Source: three-view drawing plus pictorial views. Frame: mm from the lowest corner of the part. Round coordinates to 2 decimals unless told otherwise and drop trailing zeros. Write each loop counter-clockwise with the first axis right and the second up, starting at its lowest first coordinate (ties: lowest second). Pieces come first, ordered by that corner, then holes. Notation, with made-up numbers: M 31.5,42 L 61.5,42 A21 ccw 61.5,54 Z; hole C 4,7.5 d4. An arc over 180 degrees is marked long. Put each result on its own line as item: value. Start each with the question number.
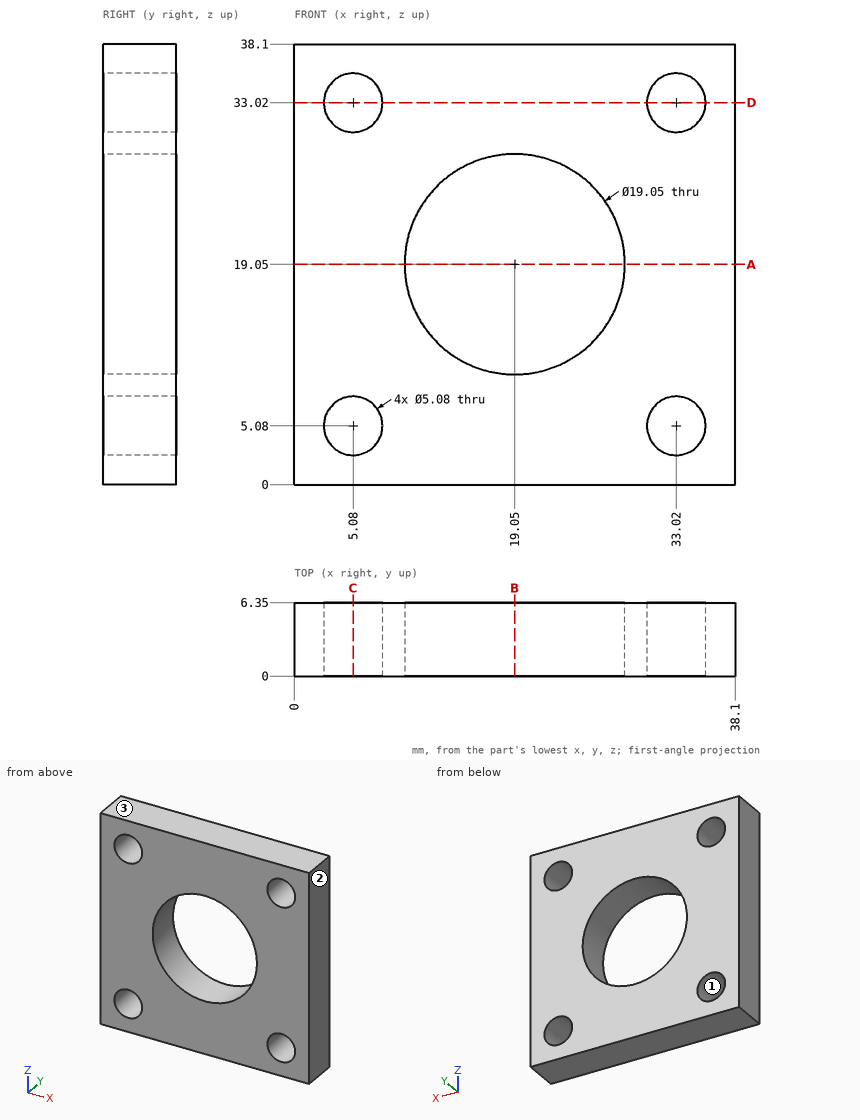
(1) Section query B-B (x = 19.05). Return loops of the section in (y, z) (3 decimals).
(2) Pull-direction query (X, two-part tool) for the marked faces 1, 2 and 3; classes: +X half, -X half, draft (parallel to the pull), parting line (faces both ways), or undercut.
(3) Section query C-C (x = 5.08). Return loops of the section in (y, z), and give its area (3 significant figures).
(4) Contact query for a flat-ended pin moving along its axis: P1, Ø8, axis at x = 16, z = 18, coming from the +Y side. Output: stop coordinate, or through.
(5) Ray query, line 1 along Z through (x, y) = (5.08, 3.75); line 2 along X through (y, z) = (1, 19.5). Return the intervals inside material, ascending.
(6) Section query A-A (z = 19.05). Return loops of the section in (x, y) (3 decimals), and give its area (3 significant figures).
(7) Section query D-D (z = 33.02). Return loops of the section in (x, y), and give its area (3 significant figures).
Entries:
1. outline: M 0,0 L 6.35,0 L 6.35,9.525 L 0,9.525 Z; M 0,28.575 L 6.35,28.575 L 6.35,38.1 L 0,38.1 Z
2. face 1: undercut
2. face 2: +X half
2. face 3: draft
3. outline: M 0,0 L 6.35,0 L 6.35,2.54 L 0,2.54 Z; M 0,7.62 L 6.35,7.62 L 6.35,30.48 L 0,30.48 Z; M 0,35.56 L 6.35,35.56 L 6.35,38.1 L 0,38.1 Z
3. area: 177 mm2
4. P1: through
5. line 1: 0 to 2.54, 7.62 to 30.48, 35.56 to 38.1
5. line 2: 0 to 9.54, 28.56 to 38.1
6. outline: M 0,0 L 9.525,0 L 9.525,6.35 L 0,6.35 Z; M 28.575,0 L 38.1,0 L 38.1,6.35 L 28.575,6.35 Z
6. area: 121 mm2
7. outline: M 0,0 L 2.54,0 L 2.54,6.35 L 0,6.35 Z; M 7.62,0 L 30.48,0 L 30.48,6.35 L 7.62,6.35 Z; M 35.56,0 L 38.1,0 L 38.1,6.35 L 35.56,6.35 Z
7. area: 177 mm2
